Geometry check sheet. Reference: the model listing, model coordinates, mm. Round coordinates to 2 decimals unless told otherwise and drop trailing zeros. Order: outer loops, then holes, each group sorted by start corner. A loop starts at its lowest first (then second) coordinate and runs counter-clockwise, first axis right, second up. Notation, with made-up numbers: M 80,11.25 L 130,11.25 A21 cw 130,29.25 Z; hole C 85.5,-1.5 d1. An arc over 180 degrees is marked long. Return JSON: item names as keys, results as strings. Group by question number.
```python
from build123d import *

# Parameters (mm, degrees)
SKETCH1_R           = 88.9
BOSS_EXTRUDE1_DEPTH = 9.525
SKETCH2_R           = 45.72
CUT_EXTRUDE1_DEPTH  = 12.7
SKETCH3_R           = 1.397
CUT_EXTRUDE2_DEPTH  = 12.7
CIRPATTERN1_COUNT   = 12
SKETCH4_R           = 1.905
CUT_EXTRUDE3_DEPTH  = 12.7
CIRPATTERN2_COUNT   = 4
SKETCH10_R          = 0.6985
CUT_EXTRUDE5_DEPTH  = 3.175
CIRPATTERN5_COUNT   = 4


with BuildPart() as part:
    # Sketch1 → Boss-Extrude1 (new body)
    with BuildSketch(Plane(origin=(0, 0, 0), x_dir=(1, 0, 0), z_dir=(0, 1, 0))):
        Circle(SKETCH1_R)
    extrude(amount=BOSS_EXTRUDE1_DEPTH)

    # Sketch2 → Cut-Extrude1 (cut)
    with BuildSketch(Plane(origin=(0, 9.525, 0), x_dir=(1, 0, 0), z_dir=(0, 1, 0))):
        Circle(SKETCH2_R)
    extrude(amount=-CUT_EXTRUDE1_DEPTH, mode=Mode.SUBTRACT)

    # Sketch3 → Cut-Extrude2 (cut)
    with BuildSketch(Plane(origin=(0, 9.525, 0), x_dir=(1, 0, 0), z_dir=(0, 1, 0))):
        with Locations((0, 51.6382)):
            Circle(SKETCH3_R)
    cut_extrude2 = extrude(amount=-CUT_EXTRUDE2_DEPTH, mode=Mode.SUBTRACT)

    # CirPattern1: Cut-Extrude2 ×12 about axis
    cirpattern1_axis = Axis((0, 0, 0), (0, 1, 0))
    for i in range(1, CIRPATTERN1_COUNT):
        add(cut_extrude2.rotate(cirpattern1_axis, i * 360 / CIRPATTERN1_COUNT), mode=Mode.SUBTRACT)

    # Sketch4 → Cut-Extrude3 (cut)
    with BuildSketch(Plane(origin=(0, 9.525, 0), x_dir=(1, 0, 0), z_dir=(0, 1, 0))):
        with Locations((0, 82.55)):
            Circle(SKETCH4_R)
    cut_extrude3 = extrude(amount=-CUT_EXTRUDE3_DEPTH, mode=Mode.SUBTRACT)

    # CirPattern2: Cut-Extrude3 ×4 about axis
    cirpattern2_axis = Axis((0, 0, 0), (0, 1, 0))
    for i in range(1, CIRPATTERN2_COUNT):
        add(cut_extrude3.rotate(cirpattern2_axis, i * 360 / CIRPATTERN2_COUNT), mode=Mode.SUBTRACT)

    # Sketch10 → Cut-Extrude5 (cut)
    with BuildSketch(Plane(origin=(-62.861792847, 0, -62.861792847), x_dir=(0, -1, 0), z_dir=(-0.707106781, 0, -0.707106781))):
        with Locations((-4.826, 0)):
            Circle(SKETCH10_R)
    cut_extrude5 = extrude(amount=-CUT_EXTRUDE5_DEPTH, mode=Mode.SUBTRACT)

    # CirPattern5: Cut-Extrude5 ×4 about axis
    cirpattern5_axis = Axis((0, 0, 0), (0, 1, 0))
    for i in range(1, CIRPATTERN5_COUNT):
        add(cut_extrude5.rotate(cirpattern5_axis, i * 360 / CIRPATTERN5_COUNT), mode=Mode.SUBTRACT)


solid = part.part
```
Q1. Section check C-C on x = 67.5. Record the cut outline in (y, z) (3 decimals).
Q2. Release check for a two-part mould opening along Z. For faces 1 (the face through (84.795, 4.696, -26.703)), 2 (the face through (-41, 0, -21)), 3 (the face through (43.61, 4.83, -13.73)) record: +Z half, -Z half, draft (parallel to the pull), parting line (faces both ways), or undercut.
Q3. Section check A-A on y = 2.5. Count the separate pieces of the cut face and the enclosed holes in it, plus the area to 3 significant figures.
Q4. Depth check by flat-ended pin: pin 1 Ø1.5 at (y, z) = (3, -23) entering from +X; pin 2 Ø4 at (y, z) = (2, -26) entering from -X; pin 3 Ø1.5 at (x, y) = (-18, 7) entering from +Z. Enter the tip coordinate at first touch or a pass-through.
Q5. Section check D-D on x = -78. Record the cut outline in (y, z) (3 decimals), plus the area to 3 significant figures.
Q6. Section check B-B on x = 14. Record the cut outline in (y, z) (3 decimals).
Q7. Material ranges on line 1 along Z through (x, y) = (0, 3.75) (3 decimals); line 2 along Z through (x, y) = (82, 5.5); line 3 along Z through (x, y) = (14.5, 5.5), recorded low to high.
Geometry check:
{
 "1": {"outline": "M 0,-57.853 L 9.525,-57.853 L 9.525,57.853 L 0,57.853 Z"},
 "2": {"face 1": "parting line", "face 2": "draft", "face 3": "undercut"},
 "3": {"separate pieces": "1", "enclosed holes": "17", "area": "18,100 mm^2"},
 "4": {"pin 1": "stops at x = 86.07", "pin 2": "stops at x = -85.6", "pin 3": "stops at z = 87.21"},
 "5": {"outline": "M 0,-42.652 L 9.525,-42.652 L 9.525,42.652 L 0,42.652 Z", "area": "813 mm^2"},
 "6": {"outline": "M 0,-87.791 L 9.525,-87.791 L 9.525,-43.524 L 0,-43.524 Z; M 0,43.524 L 9.525,43.524 L 9.525,87.791 L 0,87.791 Z"},
 "7": {"line 1": "z = -88.9 to -84.455, -80.645 to -53.035, -50.241 to -45.72, 45.72 to 50.241, 53.035 to 80.645, 84.455 to 88.9", "line 2": "z = -34.34 to -1.82, 1.82 to 34.34", "line 3": "z = -87.71 to -43.36, 43.36 to 87.71"}
}
